Autodesk Inventor part; units mm, degrees
ref_plane "Work Plane1" through (33.575, 0, 0) normal (0, 0, -1) x (1, 0, 0)
ref_plane "YZ Plane" through (0, 0, 0) normal (1, 0, 0) x (0, 1, 0)
ref_plane "XZ Plane" through (0, 0, 0) normal (0, 1, 0) x (-1, 0, 0)
sketch "Szkic1" plane through (0, 0, 0) normal (0, 0, 1) x (1, 0, 0)
  line L0 (0, 0) -> (35, 0)
  line L1 (35, 0) -> (35, 2)
  line L2 (35, 2) -> (4.1, 2)
  line L3 (4.1, 2) -> (3.6706, 1.5706)
  line L4 (3.6706, 1.5706) -> (3.1294, 1.5706)
  line L5 (3.1294, 1.5706) -> (0.5, 4.2)
  line L6 (0.5, 4.2) -> (0, 4.2)
  line L7 (0, 4.2) -> (0, 0)
  line L8 (4.1, 2) -> (2.7, 2) construction
  line L9 (-7, 0) -> (42, 0)
  line L10 (0, 5.04) -> (0, -0.84)
  dimension "d0" = 35
  dimension "d1" = 45
  dimension "d2" = 0.4294
  dimension "d3" = 30.9
  dimension "d4" = 2.7
  dimension "d5" = 3.1412
  dimension "d6" = 4
  dimension "d7" = 8.4
revolve "Bryła" add sketch "Szkic1" angle 360 about axis through (0, 0, 0) along (1, 0, 0)
sketch "Szkic2" plane through (0, 0, 0) normal (-1, 0, 0) x (0, 0, 1)
  line L0 (4.2, -0.755) -> (-4.2, -0.755)
  line L1 (-4.2, -0.755) -> (-4.2, 0.755)
  line L2 (-4.2, 0.755) -> (4.2, 0.755)
  line L3 (4.2, 0.755) -> (4.2, -0.755)
  line L4 (0, 0.755) -> (0, -0.755) construction
  line L5 (-4.2, 0) -> (4.2, 0) construction
  line L6 (0, 4.2) -> (0, 0)
  dimension "d15" = 1.51
  dimension "d16" = 8.4
extrude "Szczelina" cut sketch "Szkic2" against normal blind 1.3
thread "Gwint"
chamfer "Faza1" distance 0.4294 distance2 0.2147 1 edges at (35, -2, 0) measured on face at (35, 0.6473, -0.1595)
ref_plane "Work Plane1" through (33.575, 0, 0) normal (0, 0, -1) x (1, 0, 0)
equation "\"d0\" = NLG"
equation "\"d1\" = 0.5 * SEWI"
equation "\"d2\" = GAL"
equation "\"d3\" = GEL"
equation "\"d4\" = KOH"
equation "\"d5\" = BDM"
equation "\"d6\" = GD"
equation "\"d7\" = KOD"
equation "\"d15\" = SBR"
equation "\"d16\" = KOD"
equation "\"d8\" = STI"
equation "\"d10\" = GEL"
equation "\"d12\" = -0.5 * SPD + 0.5 * GD"
equation "\"d13\" = 0.5 * GAL"
equation "\"NLG\" = 35"
equation "\"GAL\" = 0.61345 * PTC"
equation "\"GEL\" = 30.9"
equation "\"KOH\" = 2.7"
equation "\"KOD\" = 8.4"
equation "\"SEWI\" = 90deg"
equation "\"BDM\" = NND - 1.2269 * PTC"
equation "\"GD\" = NND"
equation "\"SBR\" = 1.51"
equation "\"STI\" = 1.3"
equation "\"SPD\" = NND - 1.2269 * PTC"
equation "\"GUL\" = 0.61345 * PTC"
equation "\"PTC\" = 0.7"
equation "\"EPV\" = 4.7"
equation "\"THREADDIA\" = 4"
equation "\"TOA\" = 30deg"
equation "\"NND\" = 4"
equation "\"GD1\" = THREADDIA - 1.2269 * PTC"
properties part number "ISO 2009 - M4 x 35" material "Stal nierdzewna 440C"
Can you work these out from the model? Positions are in its coordinate system, mm. A direction names the side the tool comes from. Give positions to 0.01 mm unless a question says otherwise; leave off trailing zeros. Order: outer loops, then holes, each group sorted by start corner. A loop starts at its lowest first (then second) coordinate and runs counter-clockwise, first axis right, second up. Notation, with made-up numbers: M -11,30 L 0,30 A5 cw 0,34 Z; hole C -25,75 d9. An arc over 180 degrees is marked long. Write item = value, one per line. Start each with the question number.
Q1. For faces 4 (the flat face through (0, 2, 0)), 5 (the flat face through (1, -0.755, 0)), which set-ups out of +Z, -Z, +X, -X, +Y, -Y let a thin tool reach every point of the face, with its end or its side?
Q2. Suppose I cut it at B-B (z = 0). Write out the boundary of the cut face in (x, y) (3 decimals), plus the area to 3 significant figures.
Q3. We'd pull the mould along X, two halves only. Please class faces 1 (the flat face through (1.3, 0, 0)), 2 (the cylindrical face through (19, 0, 2)), 3 (the cylindrical face through (3.4, -1.57, -0.07)): pulls with the +X half, pulls with the -X half, needs draft (parallel to the pull), parting line crosses it, or undercut.
Q4. I need wall thicknesses on probe 1 along X at (y, z) = (2, 2.75); probe 2 along X at (y, z) = (0, 1.5); probe 3 along Z at (x, y) = (11, 0). Which ranges of each line are inside material? Lowest first, please. Write a range as [from, to].
Q5. Suppose I cut it at C-C (x = 29). Write out the boundary of the cut face in (y, z).
Q6. Will these pins go through, and if not, where does the flat tip stop? pin 1 Ø1.5 at (x, z) = (19, -0.5) entering from -Y; pin 2 Ø1.4 at (x, z) = (0.5, -1.5) entering from -Y; pin 3 Ø4 at (x, z) = (28, -1.5) entering from +Y.
Q7. Suppose I cut it at A-A (y = 0). Write out the boundary of the cut face in (x, z).
Check result:
q1.face_4 = +Z, -Z, -X, +Y, -Y
q1.face_5 = +Z, -Z, -X
q2.outline = M 0,-4.2 L 0.5,-4.2 L 3.129,-1.571 L 3.671,-1.571 L 4.1,-2 L 34.785,-2 L 35,-1.571 L 35,1.571 L 34.785,2 L 4.1,2 L 3.671,1.571 L 3.129,1.571 L 0.5,4.2 L 0,4.2 L 0,0.755 L 1.3,0.755 L 1.3,-0.755 L 0,-0.755 Z
q2.area = 144 mm2
q3.face_1 = pulls with the -X half
q3.face_2 = needs draft
q3.face_3 = undercut
q4.probe_1 = [0, 1.3]
q4.probe_2 = [1.3, 35]
q4.probe_3 = [-2, 2]
q5.outline = C 0,0 d4
q6.pin_1 = -2
q6.pin_2 = -4.12
q6.pin_3 = 2
q7.outline = M 1.3,-3.4 L 3.13,-1.57 L 3.67,-1.57 L 4.1,-2 L 34.79,-2 L 35,-1.57 L 35,1.57 L 34.79,2 L 4.1,2 L 3.67,1.57 L 3.13,1.57 L 1.3,3.4 Z
